from build123d import *

# Parameters (mm, degrees)
AUFSATZ_LINEAR_AUSTRAGEN1_DEPTH = 3
SKIZZE3_R                       = 2.5
SCHNITT_LINEAR_AUSTRAGEN1_DEPTH = 3
SKIZZE6_R                       = 2
SCHNITT_LINEAR_AUSTRAGEN3_DEPTH = 3
FILLET1_R                       = 1


with BuildPart() as part:
    # Skizze1 → Aufsatz-Linear austragen1 (new body)
    with BuildSketch(Plane.XY):
        Polygon((-37.552187815, 28), (-43.552187815, 28), (-43.552187815, 0), (-37.552187815, 0), (37.552187815, 0), (43.552187815, 0), (43.552187815, 28), (37.552187815, 28), align=None)
    extrude(amount=AUFSATZ_LINEAR_AUSTRAGEN1_DEPTH)

    # Skizze3 → Schnitt-Linear austragen1 (cut)
    with BuildSketch(Plane.XY.offset(3)):
        with Locations((-37.552187815, 12)):
            Circle(SKIZZE3_R)
        with Locations((37.552187815, 12)):
            Circle(SKIZZE3_R)
    extrude(amount=-SCHNITT_LINEAR_AUSTRAGEN1_DEPTH, mode=Mode.SUBTRACT)

    # Skizze6 → Schnitt-Linear austragen3 (cut)
    with BuildSketch(Plane.XY.offset(3)):
        with Locations((-24, 14)):
            Circle(SKIZZE6_R)
        with Locations((24, 14)):
            Circle(SKIZZE6_R)
    extrude(amount=-SCHNITT_LINEAR_AUSTRAGEN3_DEPTH, mode=Mode.SUBTRACT)

    # Fillet1
    fillet1_edges = [part.edges().sort_by_distance(p)[0] for p in [
        (-43.552187815, 14, 0),
        (-43.552187815, 14, 3),
        (43.552187815, 28, 1.5),
        (43.552187815, 0, 1.5),
        (-43.552187815, 0, 1.5),
        (-43.552187815, 28, 1.5),
        (0, 0, 3),
        (43.552187815, 14, 3),
        (0, 28, 3),
        (0, 28, 0),
        (43.552187815, 14, 0),
        (0, 0, 0),
    ]]
    fillet(fillet1_edges, radius=FILLET1_R)


solid = part.part
Verification items for the finished model (mm, model axes). Give positions to 0.01 mm unless a question says otherwise; leave off trailing zeros. Write each loop counter-clockwise with the first axis right and the second up, starting at its lowest first coordinate (ties: lowest second). Pieces come first, ordered by that corner, then holes. Notation, with made-up numbers: (-26.75, 11) -> (-15.75, 11) arc R20 ccw to (-15.75, 16) -> close; hole circle Ø6 at (77, 49). An arc over 180 degrees is marked (long way). Use CSV: the item, a comma, the result in double quotes.
(1) Release check for a two-part mould opening along X. For faces 1 (the cylindrical face through (38.706, 9.782, 1.521)), 2 (the flat face through (-1, 14, 0)) record: +X half, -X half, draft (parallel to the pull), parting line (faces both ways), or undercut.
Derived:
face 1,"undercut"
face 2,"draft"
(2) Material ranges on L1, parallel to Y at x = 24, z = 0.95; L2, parallel to Y at x = -24, z = 2.4; L3, parallel to X at y = 13, z = 2.65, recorded low to high.
Derived:
L1,"y = 0 to 12, 16 to 28"
L2,"y = 0.08 to 12, 16 to 27.92"
L3,"x = -43.31 to -39.84, -35.26 to -25.73, -22.27 to 22.27, 25.73 to 35.26, 39.84 to 43.31"
(3) Sectioned sample at A-A (x = 24). Record the cut outline in (y, z), plus the area to 3 significant figures.
Derived:
outline,"(0, 1) arc R1 ccw to (1, 0) -> (12, 0) -> (12, 3) -> (1, 3) arc R1 ccw to (0, 2) -> close; (16, 0) -> (27, 0) arc R1 ccw to (28, 1) -> (28, 2) arc R1 ccw to (27, 3) -> (16, 3) -> close"
area,"71.1 mm^2"
(4) Go/stop test with a flat-tipped pin: pin 1 (4 mm diameter, centred on x = -23, y = 14.5, fed in from +Z). Record where the tip stops, or that it passes through.
Derived:
pin 1,"stops at z = 3"
(5) Sectioned sample at C-C (x = -23). Record the cut outline in (y, z).
Derived:
outline,"(0, 1) arc R1 ccw to (1, 0) -> (12.27, 0) -> (12.27, 3) -> (1, 3) arc R1 ccw to (0, 2) -> close; (15.73, 0) -> (27, 0) arc R1 ccw to (28, 1) -> (28, 2) arc R1 ccw to (27, 3) -> (15.73, 3) -> close"
(6) Sectioned sample at B-B (y = 10.25). Record the cut outline in (x, z), plus the area to 3 significant figures.
Derived:
outline,"(-43.55, 1) arc R1 ccw to (-42.55, 0) -> (-39.34, 0) -> (-39.34, 3) -> (-42.55, 3) arc R1 ccw to (-43.55, 2) -> close; (-35.77, 0) -> (35.77, 0) -> (35.77, 3) -> (-35.77, 3) -> close; (39.34, 0) -> (42.55, 0) arc R1 ccw to (43.55, 1) -> (43.55, 2) arc R1 ccw to (42.55, 3) -> (39.34, 3) -> close"
area,"239 mm^2"
